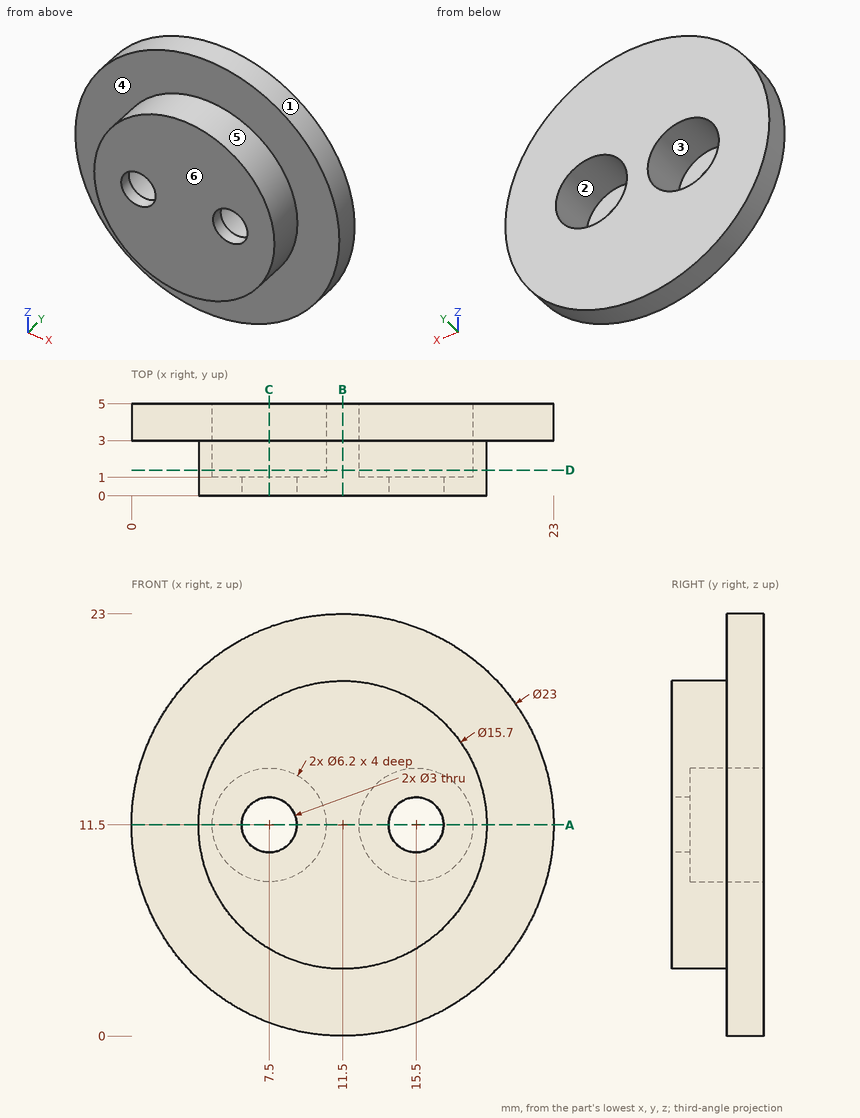
Geometry check sheet. Reference: drawing and pictorial views, mm from the part's lowest x, y, z. A direction names the side the tool comes from. Give positions to 0.01 mm unless a question says otherwise; leave off trailing zeros. Loops run counter-clockwise (first coordinate to the right, second up) from the corner with the lowest first, then second, coordinate; pieces in that order, holes last. Notation, with made-up numbers: (-20.75, 34) - (17.25, 34) arc R27 ccw to (17.25, 70) - close; hole circle Ø5 at (-4, 87.5). An arc over 180 degrees is marked (long way). One line per question, with ' | ' between items. Start each with the question number.
1. Material ranges on line 1 along X through (y, z) = (0.7, 11.5); line 2 along X through (y, z) = (3.8, 11.5); line 3 along Y through (x, z) = (3.5, 18), recorded low to high. Write a range as [from, to].
2. Cross-section at C-C, the plane x = 7.5. Enter the section's corners in (y, z).
3. Cross-section at A-A, the plane z = 11.5. Enter the section's corners in (x, y), plus the area to 3 significant figures.
4. Gauge pin test, flat ends, axial feed: pin 1 Ø4 at (x, z) = (7.5, 11.5) entering from +Y; pin 2 Ø1.5 at (y, z) = (3, 20.5) entering from -X. Record the tip position at first contact, or that the pin passes through.
5. Cross-section at B-B, the plane x = 11.5. Enter the section's corners in (y, z), plus the area to 3 significant figures.
6. Draft check along X on the marked faces 1, 2, 3 and 4. Enter one of: released by +X, released by -X, zero draft, split by the parting line, or undercut.
7. Cross-section at D-D, the plane y = 1.4. Enter the section's corners in (x, z).
8. Set-up check for the marked faces 5 and 6: record each of +Z, -Z, +X, -X, +Y, -Y from which the full face is reachable in a straight line by a thin tool's end or side.
Check result:
1) line 1: x = [3.65, 6], [9, 14], [17, 19.35] | line 2: x = [0, 4.4], [10.6, 12.4], [18.6, 23] | line 3: y = [3, 5]
2) outline: (0, 4.75) - (3, 4.75) - (3, 0.72) - (5, 0.72) - (5, 8.4) - (1, 8.4) - (1, 10) - (0, 10) - close; (0, 13) - (1, 13) - (1, 14.6) - (5, 14.6) - (5, 22.28) - (3, 22.28) - (3, 18.25) - (0, 18.25) - close
3) outline: (0, 3) - (3.65, 3) - (3.65, 0) - (6, 0) - (6, 1) - (4.4, 1) - (4.4, 5) - (0, 5) - close; (9, 0) - (14, 0) - (14, 1) - (12.4, 1) - (12.4, 5) - (10.6, 5) - (10.6, 1) - (9, 1) - close; (17, 0) - (19.35, 0) - (19.35, 3) - (23, 3) - (23, 5) - (18.6, 5) - (18.6, 1) - (17, 1) - close | area: 37.5 mm2
4) pin 1: stops at y = 1 | pin 2: stops at x = 3.49
5) outline: (0, 3.65) - (3, 3.65) - (3, 0) - (5, 0) - (5, 23) - (3, 23) - (3, 19.35) - (0, 19.35) - close | area: 93.1 mm2
6) face 1: split by the parting line | face 2: undercut | face 3: undercut | face 4: zero draft
7) outline: circle Ø15.7 at (11.5, 11.5); hole circle Ø6.2 at (7.5, 11.5); hole circle Ø6.2 at (15.5, 11.5)
8) face 5: -Y | face 6: +Z, -Z, +X, -X, -Y
